Autodesk Fusion 360 part; units mm, degrees
sketch "Sketch1" plane through (0, 0, 0) normal (0, 0, 1) x (1, 0, 0)
  line L0 (35, 20) -> (-35, 20)
  line L1 (-35, 20) -> (-35, -20)
  line L2 (-35, -20) -> (35, -20)
  line L3 (35, -20) -> (35, 20)
  line L4 (0, -20) -> (-5, -20)
  line L5 (0, -20) -> (5, -20)
  line L6 (35, 20) -> (35, 15)
  line L7 (35, 15) -> (35, 10)
  line L8 (35, 10) -> (5, -20)
  line L9 (35, 20) -> (-5, -20)
  line L10 (-35, -7.5) -> (7.5, -7.5)
  line L11 (-35, 7.5) -> (22.5, 7.5)
  dimension "d8" = 70
  dimension "d9" = 40
  dimension "d14" = 5
  dimension "d15" = 5
  dimension "d16" = 5
  dimension "d17" = 5
extrude "Extrude1" add sketch "Sketch1" along normal blind 10 contours L2 L3 L4 L5 L6 L7 L8 L9
extrude "Extrude2" add sketch "Sketch1" along normal blind 40 contours L0 L1 L9 L11 | L1 L2 L9 L10
extrude "Extrude3" add sketch "Sketch1" along normal blind 15 contours L2 L3 L8
extrude "Extrude4" add sketch "Sketch1" along normal blind 20 contours L1 L9 L10 L11
The listing builds one solid part. Answer for the finished solid, in the listing's coordinates (mm). A direction names the side the tool comes from. Give positions to 0.01 mm unless a question says otherwise; leave off trailing zeros. Write each loop counter-clockwise with the first axis right and the second up, starting at its lowest first coordinate (ties: lowest second). Pieces come first, ordered by that corner, then holes.
Item 1: Determine the mould class of faces 1 (the flat face through (20, -5, 12)), 2 (the flat face through (-8, -20, 15)), 3 (the flat face through (-35, 0.3, 19.7)), 4 (the flat face through (16, -3, 10)) for opening direction Y: released by +Y, released by -Y, zero draft, split by the parting line, or undercut.
Item 2: Find the intervals of material crossed by line 1 along Z through (x, y) = (10.5, 4); line 2 along Z through (x, y) = (24.5, -3); line 3 along Y through (x, z) = (-4.5, 32.5), in increasing order.
Item 3: Section D-D, the plane y = -3.5 is taken. Write down the section's boundary in (x, z).
Item 4: Section B-B, the plane z = 30.5 is taken. Write down the section's boundary in (x, y).
Item 5: Flat-ended cylindrical pins translate along their axes: P1, Ø7.5, axis at x = 3, y = 3, coming from the +Z side; P2, Ø1, axis at y = 13, z = 30.5, coming from the +X side; P3, Ø10, axis at x = 8, z = 29.5, coming from the -Y side. Find the tip coordinate at first contact, or state that the pin passes through.
Item 6: Section A-A, the plane y = 3 is taken. Write down the section's boundary in (x, z).
Item 7: Which of the six approach directions +Z, -Z, +X, -X, +Y, -Y give full straight-line access (tool end or side, diameter ignored) to faces 5 (the flat face through (15, 0, 18)), 6 (the flat face through (26, -11, 15)), 7 (the flat face through (-13, 0, 20))?
Item 8: Section C-C, the plane x = 1 is taken. Write down the section's boundary in (y, z).
Completed:
1. face 1: undercut
1. face 2: released by -Y
1. face 3: zero draft
1. face 4: undercut
2. line 1: z = 0 to 20
2. line 2: z = 0 to 15
2. line 3: y = -19.5 to -7.5, 7.5 to 20
3. outline: (-35, 0) - (35, 0) - (35, 15) - (21.5, 15) - (21.5, 10) - (11.5, 10) - (11.5, 20) - (-35, 20) - close
4. outline: (-35, -20) - (-5, -20) - (7.5, -7.5) - (-35, -7.5) - close; (-35, 7.5) - (22.5, 7.5) - (35, 20) - (-35, 20) - close
5. P1: stops at z = 20
5. P2: stops at x = 28.5
5. P3: stops at y = -12
6. outline: (-35, 0) - (35, 0) - (35, 15) - (28, 15) - (28, 10) - (18, 10) - (18, 20) - (-35, 20) - close
7. face 5: +Z
7. face 6: +Z, +X, -Y
7. face 7: +Z, +X, -X
8. outline: (-20, 0) - (20, 0) - (20, 40) - (7.5, 40) - (7.5, 20) - (-7.5, 20) - (-7.5, 40) - (-14, 40) - (-14, 10) - (-20, 10) - close
